Design review of the part built by this model. Coordinates are the model's own, in mm. A direction names the side the tool comes from. Coordinates: 2 decimals unless noted, no trailing zeros. Loops run counter-clockwise (first coordinate to the right, second up) from the corner with the lowest first, then second, coordinate; pieces in that order, holes last. Notation, with made-up numbers: (-23.75, -12.5) -> (11.25, -12.5) arc R28 ccw to (11.25, 26.5) -> close; hole circle Ø4 at (63, 9). An arc over 180 degrees is marked (long way). Use a Markdown table: item, result. Add a question column.
Q1. Draft analysis for pull direction X (two halves, no side actions). For faces 4 (the face through (-1.63, -107.32, 5.07)), 5 (the face through (0, 110, 5)), 6 (the face through (22.24, 91.983, 4.93)), 7 (the face through (25.094, 92.719, 5.07)), state which applies: pulls with the +X half, pulls with the -X half, needs draft (parallel to the pull), parting line crosses it, or undercut.
Q2. For probe 1 along Y at (x, z) = (0, 6.25); probe 2 along Y at (x, z) = (22.5, 7.75); probe 3 along Y at (x, z) = (-18.5, 1.75), list the stretches that pass through material, from the lowest coordinate up.
Q3. For faces 1 (the face through (19.5, 101, 5)), 2 (the face through (-19.5, -102, 5)), 3 (the face through (19.5, -102, 5)), list the 3-axis set-ups (+Z, -Z, +X, -X, +Y, -Y) from which the entire face can be reached by the end or side of a thin tool; tool diameter is ignored.
Q4. Clearance check with flat-ended pins moving along their axes: pin 1 Ø12 at (x, y) = (0, 100) entering from -Z; pin 2 Ø3 at (y, z) = (104, 4) entering from +X. State where each tip first meets the part, or that it passes through.
Q5. Take a section at A-A on z = 3.5. Write out the cut boundary in (x, y), plus the area to 3 significant figures.
Q6. Take a section at B-B on y = -90. Write out the cut boundary in (x, z), plus the area to 3 significant figures.
from build123d import *

# Parameters (mm, degrees)
ESBO_O1_W                = 55
ESBO_O1_H                = 190
ESBO_O1_R                = 2
RESSALTO_EXTRUS_O1_DEPTH = 10
FILETE1_R                = 8
ESBO_O3_W                = 39
ESBO_O3_H                = 15
RESSALTO_EXTRUS_O2_DEPTH = 10
ESBO_O4_R                = 7.5
CORTE_EXTRUS_O2_DEPTH    = 10
FILETE2_R                = 2


with BuildPart() as part:
    # Esboço1 → Ressalto-extrusão1 (new body)
    with BuildSketch(Plane.XY):
        Rectangle(ESBO_O1_W, ESBO_O1_H)
        with Locations((-22.5, 90)):
            Circle(ESBO_O1_R, mode=Mode.SUBTRACT)
        with Locations((22.5, 90)):
            Circle(ESBO_O1_R, mode=Mode.SUBTRACT)
        with Locations((-22.5, -90)):
            Circle(ESBO_O1_R, mode=Mode.SUBTRACT)
        with Locations((22.5, -90)):
            Circle(ESBO_O1_R, mode=Mode.SUBTRACT)
    extrude(amount=RESSALTO_EXTRUS_O1_DEPTH)

    # Filete1
    filete1_edges = [part.edges().sort_by_distance(p)[0] for p in [
        (27.5, -95, 5),
        (-27.5, -95, 5),
        (-27.5, 95, 5),
        (27.5, 95, 5),
    ]]
    fillet(filete1_edges, radius=FILETE1_R)

    # Esboço3 → Ressalto-extrusão2 (add)
    with BuildSketch(Plane.XY.offset(10)):
        with Locations((0, 102.5)):
            Rectangle(ESBO_O3_W, ESBO_O3_H)
        with Locations((0, -102.5)):
            Rectangle(ESBO_O3_W, ESBO_O3_H)
    extrude(amount=-RESSALTO_EXTRUS_O2_DEPTH)

    # Esboço4 → Corte-extrusão2 (cut)
    with BuildSketch(Plane.XY.offset(10)):
        with Locations((0, 100)):
            Circle(ESBO_O4_R)
        with Locations((0, -100)):
            Circle(ESBO_O4_R)
    extrude(amount=-CORTE_EXTRUS_O2_DEPTH, mode=Mode.SUBTRACT)

    # Filete2
    filete2_edges = [part.edges().sort_by_distance(p)[0] for p in [
        (-19.5, 110, 5),
        (19.5, 110, 5),
        (-19.5, -110, 5),
        (19.5, -110, 5),
    ]]
    fillet(filete2_edges, radius=FILETE2_R)


solid = part.part
Answer list:
| question | item | result |
|---|---|---|
| 1 | face 4 | undercut |
| 1 | face 5 | needs draft |
| 1 | face 6 | undercut |
| 1 | face 7 | pulls with the +X half |
| 2 | probe 1 | -110 to -107.5, -92.5 to 92.5, 107.5 to 110 |
| 2 | probe 2 | -94.42 to -92, -88 to 88, 92 to 94.42 |
| 2 | probe 3 | -109.73 to 109.73 |
| 3 | face 1 | +Z, -Z, +X, +Y |
| 3 | face 2 | +Z, -Z, -X, -Y |
| 3 | face 3 | +Z, -Z, +X, -Y |
| 4 | pin 1 | through |
| 4 | pin 2 | x = 19.5 |
| 5 | outline | (-27.5, -87) arc R8 ccw to (-19.5, -95) -> (-19.5, -108) arc R2 ccw to (-17.5, -110) -> (17.5, -110) arc R2 ccw to (19.5, -108) -> (19.5, -95) arc R8 ccw to (27.5, -87) -> (27.5, 87) arc R8 ccw to (19.5, 95) -> (19.5, 108) arc R2 ccw to (17.5, 110) -> (-17.5, 110) arc R2 ccw to (-19.5, 108) -> (-19.5, 95) arc R8 ccw to (-27.5, 87) -> close; hole circle Ø4 at (-22.5, -90); hole circle Ø4 at (-22.5, 90); hole circle Ø15 at (0, -100); hole circle Ø15 at (0, 100); hole circle Ø4 at (22.5, -90); hole circle Ø4 at (22.5, 90) |
| 5 | area | 11,200 mm² |
| 6 | outline | (-26.92, 0) -> (-24.5, 0) -> (-24.5, 10) -> (-26.92, 10) -> close; (-20.5, 0) -> (20.5, 0) -> (20.5, 10) -> (-20.5, 10) -> close; (24.5, 0) -> (26.92, 0) -> (26.92, 10) -> (24.5, 10) -> close |
| 6 | area | 458 mm² |
